Here's the drawing with two shaded views (mm, measured from the low corner). I have some questions. Give positions to 0.01 mm unless a question says otherwise; leave off trailing zeros. Order: outer loops, then holes, each group sorted by start corner. A loop starts at its lowest first (then second) coordinate and runs counter-clockwise, first axis right, second up. Notation, with made-up numbers: M -5,14.5 L 25,14.5 A24 ccw 25,27.5 Z; hole C -10.75,-19.5 d5. An arc over 180 degrees is marked long. One line per question, with ' | ' between items. Start each with the question number.
1) Please list where these lines run through material, in increasing order: line 1 along Y through (x, z) = (104.5, 0.8); line 2 along X through (y, z) = (87.5, 1.15); line 3 along X through (y, z) = (27, 0.85). Write a range as [from, to].
2) If we section it at A-A, the plane y = 47.5: Please give me the cut outline in (x, z).
3) If we section it at D-D, the plane z = 0.5: Please give me the cut outline in (x, y), plus the area to 3 significant figures.
4) If we section it at B-B, the plane y = 7.5: Please give me the cut outline in (x, z).
5) If we section it at C-C, the plane x = 44.5: Please give me the cut outline in (y, z), plus the area to 3 significant figures.
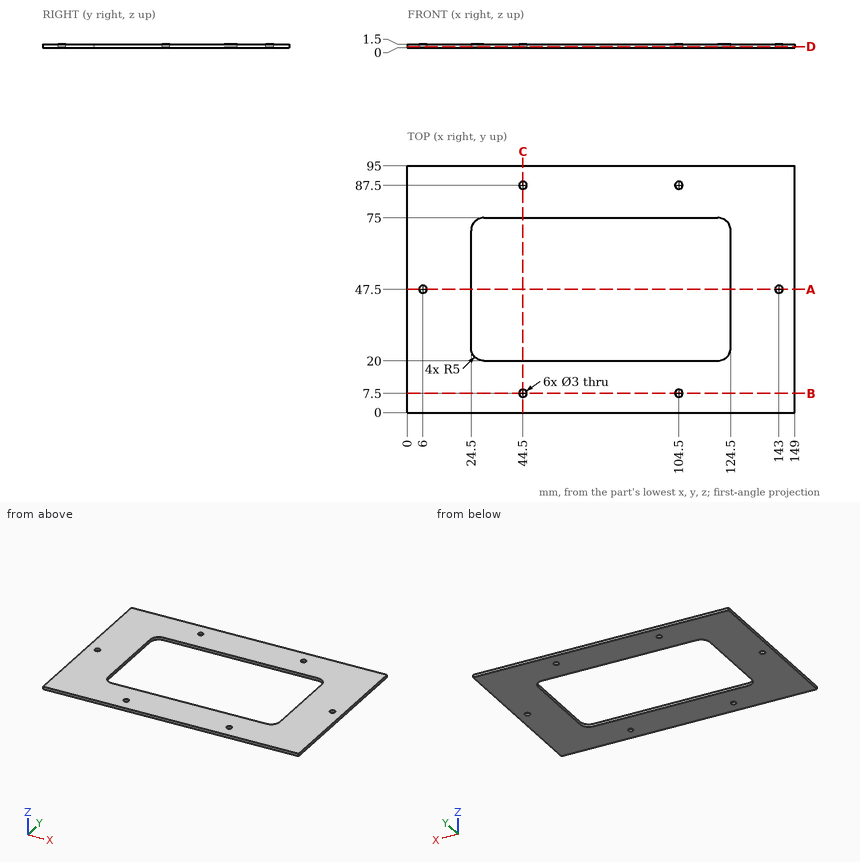
Results found:
1) line 1: y = [0, 6], [9, 20], [75, 86], [89, 95] | line 2: x = [0, 43], [46, 103], [106, 149] | line 3: x = [0, 24.5], [124.5, 149]
2) outline: M 0,0 L 4.5,0 L 4.5,1.5 L 0,1.5 Z; M 7.5,0 L 24.5,0 L 24.5,1.5 L 7.5,1.5 Z; M 124.5,0 L 141.5,0 L 141.5,1.5 L 124.5,1.5 Z; M 144.5,0 L 149,0 L 149,1.5 L 144.5,1.5 Z
3) outline: M 0,0 L 149,0 L 149,95 L 0,95 Z; hole C 6,47.5 d3; hole M 24.5,25 A5 ccw 29.5,20 L 119.5,20 A5 ccw 124.5,25 L 124.5,70 A5 ccw 119.5,75 L 29.5,75 A5 ccw 24.5,70 Z; hole C 44.5,7.5 d3; hole C 44.5,87.5 d3; hole C 104.5,7.5 d3; hole C 104.5,87.5 d3; hole C 143,47.5 d3 | area: 8,630 mm²
4) outline: M 0,0 L 43,0 L 43,1.5 L 0,1.5 Z; M 46,0 L 103,0 L 103,1.5 L 46,1.5 Z; M 106,0 L 149,0 L 149,1.5 L 106,1.5 Z
5) outline: M 0,0 L 6,0 L 6,1.5 L 0,1.5 Z; M 9,0 L 20,0 L 20,1.5 L 9,1.5 Z; M 75,0 L 86,0 L 86,1.5 L 75,1.5 Z; M 89,0 L 95,0 L 95,1.5 L 89,1.5 Z | area: 51.0 mm²
